The model under review builds one solid part; all positions refer to its coordinate system, in mm. A direction names the side the tool comes from. Coordinates: 2 decimals unless noted, no trailing zeros. Write each loop counter-clockwise with the first axis right and the second up, starting at its lowest first coordinate (ties: lowest second). Pieces come first, ordered by that corner, then holes.
1) For line 1 (X direction, y = 2.75, z = 0.8); line 2 (X direction, y = 1, z = 1.15); line 3 (X direction, y = 5, z = 1.55), list the stretches that pass through material, from the lowest coordinate up.
2) Add section B-B, the plane x = 3.25. State the section outline as (y, z) points, then the cut area to 3 significant figures.
3) Add section A-A, the plane y = -1.5. State the section outline as (x, z) points, then the cut area to 3 significant figures.
4) Add section D-D, the plane z = 0.5. State the section outline as (x, y) points, then the cut area to 3 significant figures.
5) Mouldability with a two-part tool opening along Z and no side actions: class faces 1 (the flat face through (-3.393, -2.885, -1.071)), 2 (the flat face through (-1.473, 6, 1)), 3 (the flat face through (4.728, -3.026, 0.606)), 4 (the flat face through (0, 5, -0.838)) as released by +Z, released by -Z, zero draft, split by the parting line, or undercut.
6) For P1, Ø0.6, axis at y = -1, z = -1, coming from the +X side; P2, Ø0.6, axis at x = 5, y = -0.5, coming from the +Z side; P3, Ø1, axis at x = -2.5, z = 1, coming from the -Y side, all flat-tipped, find the tip position at first contact; note any pin that passes through.
7) Machinability: for faces 5 (the flat face through (3.393, -2.885, -1.071)), 6 (the cylindrical face through (-4.67, 3.48, -1.06)), 7 (the cylindrical face through (-2.939, 5.89, 2.717)), 8 (the flat face through (-3, 1.194, 3)), 9 (the flat face through (0.965, 6, 1)), which of the approach directions +Z, -Z, +X, -X, +Y, -Y give a long, thin tool a straight path to every point of the face, cutting with its end or side? Answer none if there is none.
Autodesk Inventor part; units mm, degrees
ref_plane "Work Plane1" through (0, 1.1938, 0) normal (0, 1, 0) x (-1, 0, 0)
ref_plane "YZ Plane" through (0, 0, 0) normal (1, 0, 0) x (0, 1, 0)
ref_plane "XY Plane" through (0, 0, 0) normal (0, 0, 1) x (1, 0, 0)
ref_plane "Work Plane1" through (0, 1.1938, 0) normal (0, 1, 0) x (-1, 0, 0)
sketch "Sketch1" plane through (0, 1.1938, 0) normal (0, 1, 0) x (-1, 0, 0)
  line L0 (0, 0) -> (0, -1.3462) construction
  line L1 (3.9624, -1.3462) -> (-3.9624, -1.3462)
  line L2 (4.9784, -0.3302) -> (4.9784, 1.2192)
  line L3 (-4.9784, -0.3302) -> (-4.9784, 1.2192)
  line L4 (4.9784, 3.2258) -> (0.9652, 3.2258) construction
  line L5 (0.9652, 3.2258) -> (0.9652, 1.2192) construction
  line L6 (-4.9784, 3.2258) -> (-0.9652, 3.2258) construction
  line L7 (-0.9652, 3.2258) -> (-0.9652, 1.2192) construction
  arc A0 (4.9784, 1.2192) -> (0.9652, 1.2192) centre (2.9718, 1.2192) ccw
  arc A1 (-0.9652, 1.2192) -> (-4.9784, 1.2192) centre (-2.9718, 1.2192) ccw
  line L8 (4.9784, 1.2192) -> (4.9784, 3.2258) construction
  line L9 (-4.9784, 1.2192) -> (-4.9784, 3.2258) construction
  arc A2 (3.9624, -1.3462) -> (4.9784, -0.3302) centre (3.9624, -0.3302) ccw
  arc A3 (-4.9784, -0.3302) -> (-3.9624, -1.3462) centre (-3.9624, -0.3302) ccw
  line L10 (0.9652, 1.2192) -> (0.9652, 0)
  line L11 (-0.9652, 1.2192) -> (-0.9652, 0)
  line L12 (-1.4732, 0) -> (-1.4732, 1.2192)
  arc A4 (-1.4732, 1.2192) -> (-4.4704, 1.2192) centre (-2.9718, 1.2192) ccw
  line L13 (-4.4704, 1.2192) -> (-4.4704, -0.3302)
  arc A5 (-4.4704, -0.3302) -> (-3.9624, -0.8382) centre (-3.9624, -0.3302) ccw
  line L14 (-3.9624, -0.8382) -> (3.9624, -0.8382)
  arc A6 (3.9624, -0.8382) -> (4.4704, -0.3302) centre (3.9624, -0.3302) ccw
  line L15 (4.4704, -0.3302) -> (4.4704, 1.2192)
  arc A7 (4.4704, 1.2192) -> (1.4732, 1.2192) centre (2.9718, 1.2192) ccw
  line L16 (1.4732, 1.2192) -> (1.4732, 0)
  line L17 (1.4732, 0) -> (0.9652, 0)
  line L18 (-0.9652, 0) -> (-1.4732, 0)
  line L19 (-4.9784, 1.2192) -> (-4.4704, 1.2192)
  line L20 (4.4704, 1.2192) -> (4.9784, 1.2192)
  point P0 (4.9784, -1.3462)
  point P1 (-4.9784, -1.3462)
  dimension "d1" = 1.3462
  dimension "d2" = 9.9568
  dimension "d3" = 4.572
  dimension "d4" = 4.572
  dimension "d5" = 1.9304
  dimension "d6" = 1.016
  dimension "d7" = 0.508
extrude "Extrusion1" add sketch "Sketch1" along normal blind 9.525
extrude "Extrusion2" add sketch "Sketch1" against normal blind 5.1562 contours L1 A3 L3 L19 L13 A5 L14 A6 L15 L20 L2 A2
sketch "Sketch2" plane through (3.9624, 10.7188, -1.3462) normal (0, 0, -1) x (-1, 0, 0)
  line L0 (-0.508, 0) -> (-0.508, -14.6812) construction
  line L1 (-0.508, -14.6812) -> (-1.016, -14.1732)
  line L2 (-1.016, 0) -> (-1.016, -14.6812) construction
  line L3 (-0.508, -14.6812) -> (0.2104, -14.6812) construction
  line L4 (8.4328, 0) -> (8.4328, -14.6812) construction
  line L5 (8.4328, -14.6812) -> (8.9408, -14.1732)
  line L6 (8.9408, 0) -> (8.9408, -14.6812) construction
  line L7 (8.4328, -14.6812) -> (9.1512, -14.6812) construction
  line L8 (-0.508, -14.6812) -> (1.6764, -12.4968)
  line L9 (-0.508, -14.6812) -> (2.5812, -14.6812) construction
  line L10 (8.4328, -14.6812) -> (6.2484, -12.4968)
  line L11 (8.4328, -14.6812) -> (11.522, -14.6812) construction
  arc A0 (3.2004, -10.7188) -> (1.6764, -10.7188) centre (2.4384, -10.7188) ccw
  arc A1 (6.2484, -10.7188) -> (4.7244, -10.7188) centre (5.4864, -10.7188) ccw
  line L12 (1.6764, -12.4968) -> (1.6764, -10.7188)
  line L13 (6.2484, -12.4968) -> (6.2484, -10.7188)
  line L14 (4.7244, -10.7188) -> (3.2004, -10.7188)
  line L15 (-1.016, -14.1732) -> (-2.2198, -16.6808)
  line L16 (-2.2198, -16.6808) -> (9.9774, -16.6808)
  line L17 (9.9774, -16.6808) -> (8.9408, -14.1732)
  point P0 (3.9624, -10.7188)
  dimension "d12" = 135
  dimension "d13" = 45
  dimension "d14" = 45
  dimension "d15" = 135
  dimension "d16" = 4.572
  dimension "d17" = 1.524
  dimension "d18" = 1.524
  dimension "d19" = 0.762
  dimension "d20" = 0.762
  dimension "d21" = 0
  dimension "d22" = 0
extrude "Extrusion3" cut sketch "Sketch2" against normal through all
sketch "Sketch3" plane through (4.9784, 10.7188, 1.2192) normal (1, 0, 0) x (0, 0, -1)
  line L0 (1.5494, -14.6812) -> (2.4293, -14.6812)
  line L1 (1.5494, -14.6812) -> (0, -13.1318)
  line L2 (0, -9.525) -> (0, -14.1732)
  line L3 (1.5494, -14.6812) -> (3.7406, -14.6812) construction
  line L4 (0, -13.1318) -> (-1.4703, -15.0958)
  line L5 (1.5494, 0) -> (1.5494, -14.6812)
  line L6 (-1.4703, -15.0958) -> (1.5494, -14.6812)
  point P0 (1.2192, -10.7188)
  dimension "d25" = 135
extrude "Extrusion4" cut sketch "Sketch3" against normal through all
chamfer "Chamfer1" distance 1.2192 angle 45 2 edges at (-1.2192, 10.7188, 0) (1.2192, 10.7188, 0)
properties part number "fuse clip"
Geometry results:
1. line 1: x = -4.98 to -4.47, -1.47 to -0.97, 0.97 to 1.47, 4.47 to 4.98
1. line 2: x = -4.98 to -4.47, 4.47 to 4.98
1. line 3: x = -4.95 to -4.43, -1.51 to -0.99, 0.99 to 1.51, 4.43 to 4.95
2. outline: (-2.74, -1.35) - (10.72, -1.35) - (10.72, -0.84) - (-2.74, -0.84) - close; (1.19, 2.69) - (10.72, 2.69) - (10.72, 3.21) - (1.19, 3.21) - close
2. area: 11.7 mm2
3. outline: (-4.98, -0.33) arc R1.02 ccw to (-3.96, -1.35) - (-2.29, -1.35) - (-2.29, -0.84) - (-3.96, -0.84) arc R0.51 cw to (-4.47, -0.33) - (-4.47, 1.22) - (-4.98, 1.22) - close; (2.29, -1.35) - (3.96, -1.35) arc R1.02 ccw to (4.98, -0.33) - (4.98, 1.22) - (4.47, 1.22) - (4.47, -0.33) arc R0.51 cw to (3.96, -0.84) - (2.29, -0.84) - close
3. area: 4.49 mm2
4. outline: (-4.98, -3.13) - (-4.47, -3.13) - (-4.47, 10.72) - (-4.98, 10.72) - close; (-1.47, 1.19) - (-0.97, 1.19) - (-0.97, 10) - (-1.47, 10) - close; (0.97, 1.19) - (1.47, 1.19) - (1.47, 10) - (0.97, 10) - close; (4.47, -3.13) - (4.98, -3.13) - (4.98, 10.72) - (4.47, 10.72) - close
4. area: 23.0 mm2
5. face 1: zero draft
5. face 2: undercut
5. face 3: released by +Z
5. face 4: undercut
6. P1: stops at x = 4.91
6. P2: stops at z = 1.22
6. P3: passes through
7. face 5: +Z, -Z, -Y
7. face 6: -Z, -X, +Y, -Y
7. face 7: +Y, -Y
7. face 8: +Z, -Y
7. face 9: +Z, +Y, -Y
